Geometry check sheet. Reference: the model listing, model coordinates, mm. A direction names the side the tool comes from. Give positions to 0.01 mm unless a question says otherwise; leave off trailing zeros. Write item = value, one per line. Start each with the question number.
```python
from build123d import *

# Parameters (mm, degrees)
SKETCH_1_W           = 30
SKETCH_1_H           = 20
SKETCH_1_W_2         = 28
SKETCH_1_H_2         = 18
EXTRUDE_1_DEPTH      = 295
SKETCH_5_R           = 2.025
CUT_EXTRUDE_4_DEPTH  = 5
SKETCH_7_R           = 3.8
CUT_EXTRUDE_5_DEPTH  = 5
SKETCH_11_R          = 2.025
CUT_EXTRUDE_9_DEPTH  = 113
SKETCH_18_R          = 2.025
CUT_EXTRUDE_16_DEPTH = 90
SKETCH_21_R          = 2.025
CUT_EXTRUDE_19_DEPTH = 126
SKETCH_22_R          = 2.025
CUT_EXTRUDE_20_DEPTH = 10
SKETCH_26_R          = 1.525
CUT_EXTRUDE_24_DEPTH = 10
SKETCH_27_R          = 1.525
CUT_EXTRUDE_25_DEPTH = 100
CUT_EXTRUDE_26_DEPTH = 100
SKETCH_31_R          = 2.025
CUT_EXTRUDE_29_DEPTH = 50
SKETCH_32_R          = 3.75
CUT_EXTRUDE_30_DEPTH = 10
SKETCH_36_R          = 2.025
CUT_EXTRUDE_33_DEPTH = 37
SKETCH_37_R          = 3.8
CUT_EXTRUDE_34_DEPTH = 10


with BuildPart() as part:
    # 草图1 → 凸台-拉伸1 (new, symmetric)
    with BuildSketch(Plane.XY):
        Rectangle(SKETCH_1_W, SKETCH_1_H)
        Rectangle(SKETCH_1_W_2, SKETCH_1_H_2, mode=Mode.SUBTRACT)
    extrude(amount=EXTRUDE_1_DEPTH, both=True)

    # 草图5 → 切除-拉伸4 (cut, symmetric)
    with BuildSketch(Plane.XZ.offset(-9)):
        with Locations((-9.5, -172.5)):
            Circle(SKETCH_5_R)
        with Locations((9.5, -172.5)):
            Circle(SKETCH_5_R)
        with Locations((-9.5, -201.5)):
            Circle(SKETCH_5_R)
        with Locations((9.5, -201.5)):
            Circle(SKETCH_5_R)
        with Locations((-9.5, -14.5)):
            Circle(SKETCH_5_R)
        with Locations((9.5, -14.5)):
            Circle(SKETCH_5_R)
        with Locations((-9.5, 14.5)):
            Circle(SKETCH_5_R)
        with Locations((9.5, 14.5)):
            Circle(SKETCH_5_R)
        with Locations((-9.5, 172.5)):
            Circle(SKETCH_5_R)
        with Locations((-9.5, 201.5)):
            Circle(SKETCH_5_R)
        with Locations((9.5, 201.5)):
            Circle(SKETCH_5_R)
        with Locations((9.5, 172.5)):
            Circle(SKETCH_5_R)
    extrude(amount=CUT_EXTRUDE_4_DEPTH, both=True, mode=Mode.SUBTRACT)

    # 草图7 → 切除-拉伸5 (cut, symmetric)
    with BuildSketch(Plane(origin=(0, -9, 0), x_dir=(1, 0, 0), z_dir=(0, 1, 0))):
        with Locations((-9.5, 201.5)):
            Circle(SKETCH_7_R)
        with Locations((9.5, 201.5)):
            Circle(SKETCH_7_R)
        with Locations((-9.5, 172.5)):
            Circle(SKETCH_7_R)
        with Locations((9.5, 172.5)):
            Circle(SKETCH_7_R)
        with Locations((-9.5, 14.5)):
            Circle(SKETCH_7_R)
        with Locations((9.5, 14.5)):
            Circle(SKETCH_7_R)
        with Locations((-9.5, -14.5)):
            Circle(SKETCH_7_R)
        with Locations((9.5, -14.5)):
            Circle(SKETCH_7_R)
        with Locations((-9.5, -172.5)):
            Circle(SKETCH_7_R)
        with Locations((9.5, -172.5)):
            Circle(SKETCH_7_R)
        with Locations((-9.5, -201.5)):
            Circle(SKETCH_7_R)
        with Locations((9.5, -201.5)):
            Circle(SKETCH_7_R)
    extrude(amount=CUT_EXTRUDE_5_DEPTH, both=True, mode=Mode.SUBTRACT)

    # 草图11 → 切除-拉伸9 (cut)
    with BuildSketch(Plane(origin=(15, 0, 0), x_dir=(0, 0, -1), z_dir=(1, 0, 0))):
        with Locations((217, 0)):
            Circle(SKETCH_11_R)
        with Locations((187, 0)):
            Circle(SKETCH_11_R)
        with Locations((157, 0)):
            Circle(SKETCH_11_R)
        with Locations((30, 0)):
            Circle(SKETCH_11_R)
        Circle(SKETCH_11_R)
        with Locations((-30, 0)):
            Circle(SKETCH_11_R)
        with Locations((-157, 0)):
            Circle(SKETCH_11_R)
        with Locations((-187, 0)):
            Circle(SKETCH_11_R)
        with Locations((-217, 0)):
            Circle(SKETCH_11_R)
        with Locations((-236, 0)):
            Circle(SKETCH_11_R)
        with Locations((-260.5, 0)):
            Circle(SKETCH_11_R)
        with Locations((-285, 0)):
            Circle(SKETCH_11_R)
    extrude(amount=-CUT_EXTRUDE_9_DEPTH, mode=Mode.SUBTRACT)

    # 草图18 → 切除-拉伸16 (cut)
    with BuildSketch(Plane.XZ.offset(10)):
        with Locations((-9, 74)):
            Circle(SKETCH_18_R)
        with Locations((9, 74)):
            Circle(SKETCH_18_R)
        with Locations((-9, 56)):
            Circle(SKETCH_18_R)
        with Locations((9, 56)):
            Circle(SKETCH_18_R)
    cut_extrude_16 = extrude(amount=-CUT_EXTRUDE_16_DEPTH, mode=Mode.SUBTRACT)

    # 镜向1: 切除-拉伸16 across plane
    add(cut_extrude_16.mirror(Plane.XY), mode=Mode.SUBTRACT)

    # 草图21 → 切除-拉伸19 (cut)
    with BuildSketch(Plane(origin=(15, 0, 0), x_dir=(0, 0, -1), z_dir=(1, 0, 0))):
        with Locations((-46, 0)):
            Circle(SKETCH_21_R)
        with Locations((-84, 0)):
            Circle(SKETCH_21_R)
    extrude(amount=-CUT_EXTRUDE_19_DEPTH, mode=Mode.SUBTRACT)

    # 草图22 → 切除-拉伸20 (cut)
    with BuildSketch(Plane(origin=(0, 10, 0), x_dir=(1, 0, 0), z_dir=(0, 1, 0))):
        with Locations((-9, 285)):
            Circle(SKETCH_22_R)
        with Locations((9, 285)):
            Circle(SKETCH_22_R)
    extrude(amount=-CUT_EXTRUDE_20_DEPTH, mode=Mode.SUBTRACT)

    # 草图26 → 切除-拉伸24 (cut)
    with BuildSketch(Plane.XZ.offset(10)):
        with Locations((-11, 124)):
            Circle(SKETCH_26_R)
        with Locations((-11, 144)):
            Circle(SKETCH_26_R)
        with Locations((11, 144)):
            Circle(SKETCH_26_R)
        with Locations((11, 124)):
            Circle(SKETCH_26_R)
    extrude(amount=-CUT_EXTRUDE_24_DEPTH, mode=Mode.SUBTRACT)

    # 草图27 → 切除-拉伸25 (cut)
    with BuildSketch(Plane.ZY.offset(15)):
        with Locations((134, -6)):
            Circle(SKETCH_27_R)
        with Locations((114, -6)):
            Circle(SKETCH_27_R)
    extrude(amount=-CUT_EXTRUDE_25_DEPTH, mode=Mode.SUBTRACT)

    # 草图28 → 切除-拉伸26 (cut)
    with BuildSketch(Plane(origin=(15, 0, 0), x_dir=(0, 0, -1), z_dir=(1, 0, 0))):
        with BuildLine():
            Line((-71, 5), (-59, 5))
            ThreePointArc((-59, 5), (-54, 0), (-59, -5))
            Line((-59, -5), (-71, -5))
            ThreePointArc((-71, -5), (-76, 0), (-71, 5))
        make_face()
    cut_extrude_26 = extrude(amount=-CUT_EXTRUDE_26_DEPTH, mode=Mode.SUBTRACT)

    # 镜向2: 切除-拉伸26 across plane
    add(cut_extrude_26.mirror(Plane.XY), mode=Mode.SUBTRACT)

    # 草图31 → 切除-拉伸29 (cut)
    with BuildSketch(Plane(origin=(0, 10, 0), x_dir=(1, 0, 0), z_dir=(0, 1, 0))):
        with Locations((0, 72)):
            Circle(SKETCH_31_R)
        with Locations((0, 132)):
            Circle(SKETCH_31_R)
    extrude(amount=-CUT_EXTRUDE_29_DEPTH, mode=Mode.SUBTRACT)

    # 草图32 → 切除-拉伸30 (cut)
    with BuildSketch(Plane.ZY.offset(15)):
        with Locations((46, 0)):
            Circle(SKETCH_32_R)
        with Locations((84, 0)):
            Circle(SKETCH_32_R)
    extrude(amount=-CUT_EXTRUDE_30_DEPTH, mode=Mode.SUBTRACT)

    # 草图36 → 切除-拉伸33 (cut)
    with BuildSketch(Plane(origin=(0, 10, 0), x_dir=(1, 0, 0), z_dir=(0, 1, 0))):
        with Locations((-9, 244)):
            Circle(SKETCH_36_R)
        with Locations((-9, 216)):
            Circle(SKETCH_36_R)
        with Locations((9, 216)):
            Circle(SKETCH_36_R)
        with Locations((9, 244)):
            Circle(SKETCH_36_R)
    cut_extrude_33 = extrude(amount=-CUT_EXTRUDE_33_DEPTH, mode=Mode.SUBTRACT)

    # 草图37 → 切除-拉伸34 (cut)
    with BuildSketch(Plane.XZ.offset(10)):
        with Locations((-9, -216)):
            Circle(SKETCH_37_R)
        with Locations((9, -216)):
            Circle(SKETCH_37_R)
        with Locations((-9, -244)):
            Circle(SKETCH_37_R)
        with Locations((9, -244)):
            Circle(SKETCH_37_R)
    cut_extrude_34 = extrude(amount=-CUT_EXTRUDE_34_DEPTH, mode=Mode.SUBTRACT)

    # 镜向3: 切除-拉伸33, 切除-拉伸34 across plane
    add(cut_extrude_33.mirror(Plane.XY), mode=Mode.SUBTRACT)
    add(cut_extrude_34.mirror(Plane.XY), mode=Mode.SUBTRACT)


solid = part.part
```
1) Draft check along X on faces 3 (the flat face through (15, 0, 4)), 4 (the flat face through (-15, 0, 4)), 5 (the flat face through (14, 0, 4)), 6 (the flat face through (0, 10, 4)). Enter one of: released by +X, released by -X, zero draft, split by the parting line, or undercut.
2) Thickness scan on line 1 (X direction, y = -9.75, z = -172.5); line 2 (Y direction, x = -14.45, z = 84); line 3 (Y direction, x = 12.25, z = 226.5). Record the ranges inside material, lowest first.
3) Depth check by flat-ended pin: pin 1 Ø3 at (x, z) = (9, -216) entering from -Y; pin 2 Ø4 at (x, z) = (-11.5, 125) entering from -Y; pin 3 Ø5.5 at (x, z) = (-9.5, -14.5) entering from -Y. Enter the tip coordinate at first touch or a pass-through.
4) Tool access check on faces 1 (the flat face through (0, 9, 4)), 2 (the flat face through (-1.2, -9.6, 295)). Record the directions out of +Z, -Z, +X, -X, +Y, -Y that give a thin tool (end or side, any length) a straight path to the whole face; none if there is none.
Check result:
q1.face_3 = released by +X
q1.face_4 = released by -X
q1.face_5 = undercut
q1.face_6 = zero draft
q2.line_1 = -15 to -13.3, -5.7 to 5.7, 13.3 to 15
q2.line_2 = -10 to -3.75, 3.75 to 10
q2.line_3 = -10 to -9, 9 to 10
q3.pin_1 = through
q3.pin_2 = -10
q3.pin_3 = 9
q4.face_1 = +Z, -Z
q4.face_2 = +Z, +X, -X, +Y, -Y
